```python
from build123d import *

# Parameters (mm, degrees)
SKETCH1_W           = 25.4
SKETCH1_H           = 25.4
BOSS_EXTRUDE1_DEPTH = 2.54
BOSS_EXTRUDE2_DEPTH = 10.16
SKETCH3_R           = 1.905
CUT_EXTRUDE1_DEPTH  = 6.35


with BuildPart() as part:
    # Sketch1 → Boss-Extrude1 (new body)
    with BuildSketch(Plane(origin=(0, 0, 0), x_dir=(1, 0, 0), z_dir=(0, 1, 0))):
        with Locations((12.7, 12.7)):
            Rectangle(SKETCH1_W, SKETCH1_H)
    extrude(amount=BOSS_EXTRUDE1_DEPTH)

    # Sketch2 → Boss-Extrude2 (add)
    with BuildSketch(Plane(origin=(0, 2.54, 0), x_dir=(1, 0, 0), z_dir=(0, 1, 0))):
        Polygon((0, 25.4), (0, 0), (25.4, 0), (25.4, 6.35), (6.35, 6.35), (6.35, 25.4), align=None)
    extrude(amount=BOSS_EXTRUDE2_DEPTH)

    # Sketch3 → Cut-Extrude1 (cut)
    with BuildSketch(Plane(origin=(0, 12.7, 0), x_dir=(1, 0, 0), z_dir=(0, 1, 0))):
        with Locations((3.175, 20.32)):
            Circle(SKETCH3_R)
        with Locations((3.175, 3.175)):
            Circle(SKETCH3_R)
        with Locations((20.32, 3.175)):
            Circle(SKETCH3_R)
    extrude(amount=-CUT_EXTRUDE1_DEPTH, mode=Mode.SUBTRACT)


solid = part.part
```
Verification items for the finished model (mm, model axes). A direction names the side the tool comes from. Give positions to 0.01 mm unless a question says otherwise; leave off trailing zeros. Order: outer loops, then holes, each group sorted by start corner. A loop starts at its lowest first (then second) coordinate and runs counter-clockwise, first axis right, second up. Notation, with made-up numbers: (78, 56) - (95, 56) arc R13 cw to (95, 80) - close; hole circle Ø3 at (-3.75, 20.5). An arc over 180 degrees is marked (long way). Answer as CSV lines item,"result". Start each with the question number.
Item 1: Section check C-C, the plane x = 20.32. Record the boundary of the cut face in (y, z).
Item 2: Material ranges on L1, parallel to Z at x = 24.25, y = 11; L2, parallel to X at y = 6.5, z = -20.5; L3, parallel to Z at x = 3.75, y = 9.25, recorded low to high.
Item 3: Section check B-B, the plane y = 8.25. Record the boundary of the cut face in (x, z) (3 decimals).
Item 4: Access from +Z, -Z, +X, -X, +Y, -Y to the whole of each face (thin tool, end or side, straight path). Record for faces 4 (the face through (0, 6, -13)), 5 (the face through (16, 2.54, -16)), 6 (the face through (3, 6.35, -20)).
Item 5: Mould release check, pull along X, two halves, no side actions. Record for faces 1 (the face through (20, 6.35, -3)), 2 (the face through (13, 0, -13)), 3 (the face through (6.35, 8, -16)): released by +X, released by -X, zero draft, split by the parting line, or undercut.
Item 6: Section check A-A, the plane z = -20.32. Record the boundary of the cut face in (x, y).
Item 7: Section check D-D, the plane y = 3. Record the boundary of the cut face in (x, z), plus the area to 3 significant figures.
Item 8: Gauge pin test, flat ends, axial feed: pin 1 (9.5 mm diameter, centred on x = 17.5, z = -11.5, fed in from +Y); pin 2 (2 mm diameter, centred on x = 8.5, y = 9, fed in from -Z); pin 3 (1.9 mm diameter, centred on x = 3, z = -4, fed in from +Y). Record the tip position at first contact, or that the pin passes through.
Filled in:
1,outline,"(0, -25.4) - (2.54, -25.4) - (2.54, -6.35) - (12.7, -6.35) - (12.7, -5.08) - (6.35, -5.08) - (6.35, -1.27) - (12.7, -1.27) - (12.7, 0) - (0, 0) - close"
2,L1,"-6.35 to 0"
2,L2,"0 to 1.28, 5.07 to 6.35"
2,L3,"-25.4 to -22.14, -18.5 to -4.99, -1.36 to 0"
3,outline,"(0, -25.4) - (6.35, -25.4) - (6.35, -6.35) - (25.4, -6.35) - (25.4, 0) - (0, 0) - close; hole circle Ø3.81 at (3.175, -20.32); hole circle Ø3.81 at (3.175, -3.175); hole circle Ø3.81 at (20.32, -3.175)"
4,face 4,"+Z, -Z, -X, +Y, -Y"
4,face 5,"-Z, +X, +Y"
4,face 6,"+Y"
5,face 1,"undercut"
5,face 2,"zero draft"
5,face 3,"released by +X"
6,outline,"(0, 0) - (25.4, 0) - (25.4, 2.54) - (6.35, 2.54) - (6.35, 12.7) - (5.08, 12.7) - (5.08, 6.35) - (1.27, 6.35) - (1.27, 12.7) - (0, 12.7) - close"
7,outline,"(0, -25.4) - (6.35, -25.4) - (6.35, -6.35) - (25.4, -6.35) - (25.4, 0) - (0, 0) - close"
7,area,"282 mm^2"
8,pin 1,"y = 2.54"
8,pin 2,"z = -6.35"
8,pin 3,"y = 6.35"
